The drawing under review shows one solid part. Ordinate dimensions are in mm from its lowest x, y, z. Coordinates: 2 decimals unless noted, no trailing zeros. Order: outer loops, then holes, each group sorted by start corner. A loop starts at its lowest first (then second) coordinate and runs counter-clockwise, first axis right, second up. Notation, with made-up numbers: (87, 68.25) - (124, 68.25) arc R22 ccw to (124, 75.25) - close; hole circle Ø4 at (79, 24.25). An arc over 180 degrees is marked (long way). Answer in a Markdown table with one row per item.
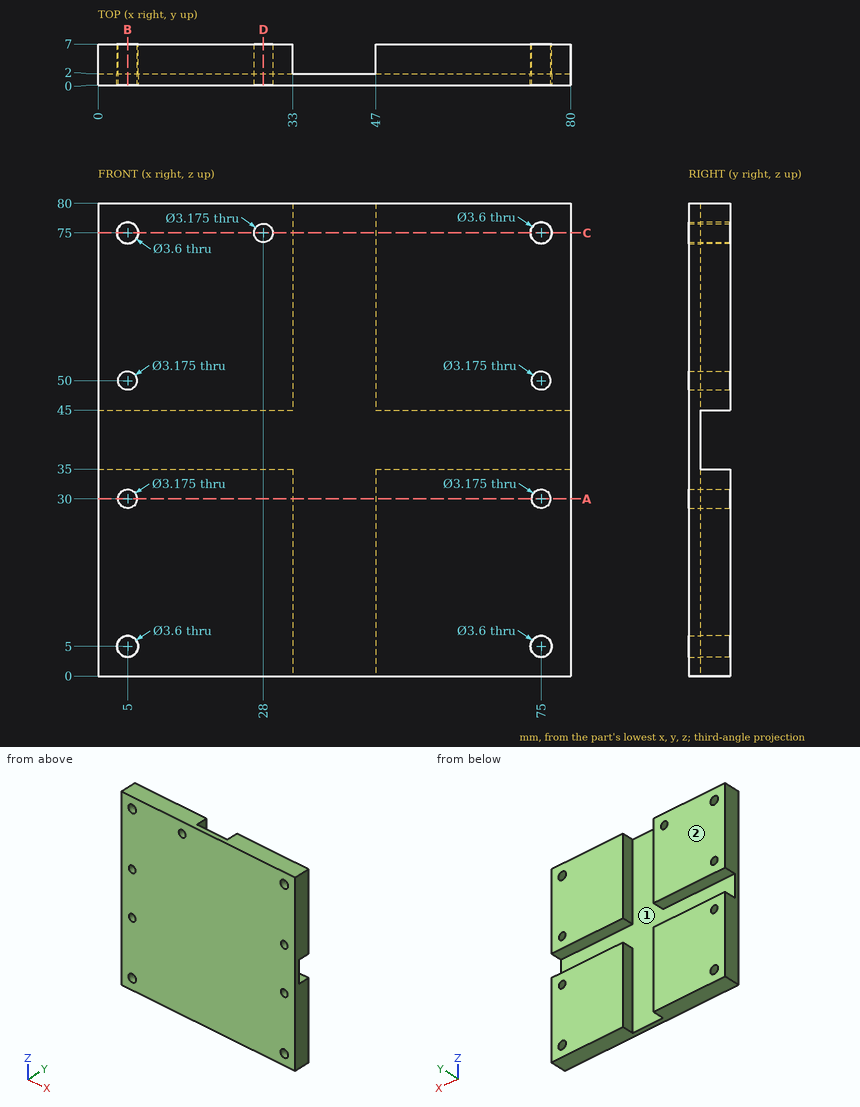
Item 1: Mouldability with a two-part tool opening along Z and no side actions: class the marked faces 1 and 2 as +Z half, -Z half, draft (parallel to the pull), parting line (faces both ways), or undercut.
Check values:
| item | result |
|---|---|
| face 1 | undercut |
| face 2 | draft |
Item 2: We need section C-C, the plane z = 75. Write out the cut boundary in (x, y), then the cut area to 3 significant figures.
Check values:
| item | result |
|---|---|
| outline | (0, 0) - (3.2, 0) - (3.2, 7) - (0, 7) - close; (6.8, 0) - (26.41, 0) - (26.41, 7) - (6.8, 7) - close; (29.59, 0) - (73.2, 0) - (73.2, 7) - (47, 7) - (47, 2) - (33, 2) - (33, 7) - (29.59, 7) - close; (76.8, 0) - (80, 0) - (80, 7) - (76.8, 7) - close |
| area | 417 mm^2 |
Item 3: We need section B-B, the plane x = 5. Write out the cut boundary in (y, z).
Check values:
| item | result |
|---|---|
| outline | (0, 0) - (7, 0) - (7, 3.2) - (0, 3.2) - close; (0, 6.8) - (7, 6.8) - (7, 28.41) - (0, 28.41) - close; (0, 31.59) - (7, 31.59) - (7, 35) - (2, 35) - (2, 45) - (7, 45) - (7, 48.41) - (0, 48.41) - close; (0, 51.59) - (7, 51.59) - (7, 73.2) - (0, 73.2) - close; (0, 76.8) - (7, 76.8) - (7, 80) - (0, 80) - close |
Item 4: We need section D-D, the plane x = 28. Write out the cut boundary in (y, z).
Check values:
| item | result |
|---|---|
| outline | (0, 0) - (7, 0) - (7, 35) - (2, 35) - (2, 45) - (7, 45) - (7, 73.41) - (0, 73.41) - close; (0, 76.59) - (7, 76.59) - (7, 80) - (0, 80) - close |
Item 5: Clearance check with a flat-ended pin moving along its axis: pin 1 Ø3 at (x, z) = (75, 75) entering from +Y. State where the tip first meets the part, or that it passes through.
Check values:
| item | result |
|---|---|
| pin 1 | through |
Item 6: To check wall thickness, follow line 1 (X direction, y = 4.1, z = 5); line 2 (Z direction, x = 75, y = 0.5); line 3 (X direction, y = 0.8, z = 75). State the ranges of each line that lie inside material, in increasing order. Write a range as from..to.
Check values:
| item | result |
|---|---|
| line 1 | 0..3.2, 6.8..33, 47..73.2, 76.8..80 |
| line 2 | 0..3.2, 6.8..28.41, 31.59..48.41, 51.59..73.2, 76.8..80 |
| line 3 | 0..3.2, 6.8..26.41, 29.59..73.2, 76.8..80 |
Item 7: We need section A-A, the plane z = 30. Write out the cut boundary in (x, y), then the cut area to 3 significant figures.
Check values:
| item | result |
|---|---|
| outline | (0, 0) - (3.41, 0) - (3.41, 7) - (0, 7) - close; (6.59, 0) - (73.41, 0) - (73.41, 7) - (47, 7) - (47, 2) - (33, 2) - (33, 7) - (6.59, 7) - close; (76.59, 0) - (80, 0) - (80, 7) - (76.59, 7) - close |
| area | 446 mm^2 |
